Work out the finished part from the listing and answer in its coordinate system (mm). Face numbers are marked on the shaded views. A direction names the side the tool comes from. Coordinates: 2 decimals unless noted, no trailing zeros. Loops run counter-clockwise (first coordinate to the right, second up) from the corner with the lowest first, then second, coordinate; pieces in that order, holes last.
```python
from build123d import *

# Parameters (mm, degrees)
SM_BASE_FLANGE_1_DEPTH = 110
FILLET_1_R             = 10


# Sheet-metal steps are written as plain solids
with BuildPart() as part:
    # Sketch 1 → 基体-法兰1 (new body)
    with BuildSketch(Plane.XY):
        with BuildLine():
            Line((0, 0), (42.015440419, -107.372792183))
            ThreePointArc((42.015440419, -107.372792183), (46.425499978, -112.91144556), (53.190353776, -115))
            Line((53.190353776, -115), (179, -115))
            ThreePointArc((179, -115), (183.242640687, -116.757359313), (185, -121))
            Line((185, -121), (185, -175))
            Line((185, -175), (191, -175))
            Line((191, -175), (191, -121))
            ThreePointArc((191, -121), (187.485281374, -112.514718626), (179, -109))
            Line((179, -109), (53.190353776, -109))
            ThreePointArc((53.190353776, -109), (49.807926877, -107.95572278), (47.602897098, -105.186396091))
            Line((47.602897098, -105.186396091), (5.587456678, 2.186396091))
            Line((5.587456678, 2.186396091), (0, 0))
        make_face()
    extrude(amount=SM_BASE_FLANGE_1_DEPTH)

    # 圆角1
    fillet_1_edges = [part.edges().sort_by_distance(p)[0] for p in [
        (188, -175, 0),
        (188, -175, 110),
    ]]
    fillet(fillet_1_edges, radius=FILLET_1_R)


solid = part.part
```
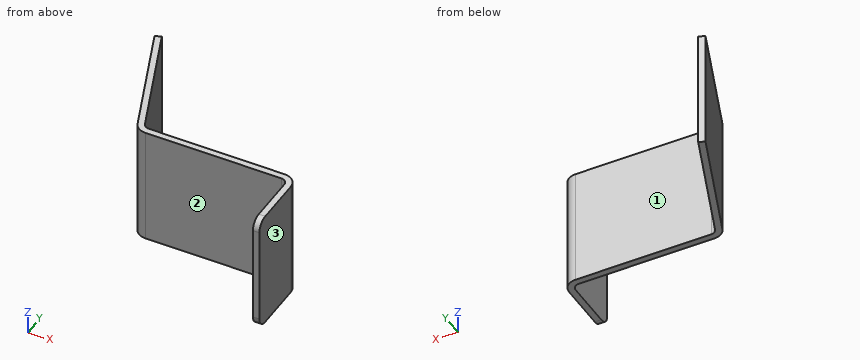
1. A cutting plane is placed at B-B, the plane y = -162. Give the vertices of the cut face in (x, z), then the cut area to 3 significant figures.
2. Each of these flat-tipped pins is pushed along its axis until it touches: P1, Ø6, axis at x = 84.5, z = 62, coming from the -Y side; P2, Ø3, axis at y = -32, z = 66.5, coming from the -X side; P3, Ø4, axis at x = 58, z = 50.5, coming from the +Y side. Where does it stop, or does it pass through?
3. A cutting plane is placed at A-A, the plane z = 64. Give the vertices of the cut face in (x, y), then the cut area to 3 significant figures.
4. Straight lines are drawn through the part: probe 1 along Y at (x, z) = (137, 55.5); probe 2 along X at (y, z) = (-142, 73.5); probe 3 along X at (y, z) = (-81, 99.5). For each, find the intervals that lie inside material, in ascending order.
5. A cutting plane is placed at C-C, the plane x = 145.5. Give the vertices of the cut face in (y, z).
6. For the marked faces 1, 2 and 3, determine the directions among +Z, -Z, +X, -X, +Y, -Y from which every point of the face is accessible in a straight line to the end or side of a thin tool.
7. A cutting plane is placed at D-D, the plane z = 7.5. Give the vertices of the cut face in (x, y).
Answers below:
1. outline: (185, 0) - (191, 0) - (191, 110) - (185, 110) - close
1. area: 660 mm2
2. P1: stops at y = -115
2. P2: stops at x = 11.93
2. P3: stops at y = -109
3. outline: (0, 0) - (42.02, -107.37) arc R12 ccw to (53.19, -115) - (179, -115) arc R6 cw to (185, -121) - (185, -175) - (191, -175) - (191, -121) arc R12 ccw to (179, -109) - (53.19, -109) arc R6 cw to (47.6, -105.19) - (5.59, 2.19) - close
3. area: 1,920 mm2
4. probe 1: y = -115 to -109
4. probe 2: x = 185 to 191
4. probe 3: x = 31.7 to 38.14
5. outline: (-115, 0) - (-109, 0) - (-109, 110) - (-115, 110) - close
6. face 1: +Z, -Z, +X, +Y
6. face 2: +Z, -Z, -X, -Y
6. face 3: +Z, -Z, +X, +Y, -Y
7. outline: (0, 0) - (42.02, -107.37) arc R12 ccw to (53.19, -115) - (179, -115) arc R6 cw to (185, -121) - (185, -174.68) - (191, -174.68) - (191, -121) arc R12 ccw to (179, -109) - (53.19, -109) arc R6 cw to (47.6, -105.19) - (5.59, 2.19) - close
